from build123d import *

# Parameters (mm, degrees)
SKETCH1_R           = 2.5
BOSS_EXTRUDE1_DEPTH = 6


with BuildPart() as part:
    # Sketch1 → Boss-Extrude1 (new body)
    with BuildSketch(Plane(origin=(0, 0, 0), x_dir=(1, 0, 0), z_dir=(0, 1, 0))):
        with BuildLine():
            Line((29.312544284, -14.726094949), (29.830902437, -13.828272291))
            ThreePointArc((29.830902437, -13.828272291), (29.893839703, -13.350216293), (29.600306432, -12.967676287))
            Line((29.600306432, -12.967676287), (7.429695757, -0.167468245))
            ThreePointArc((7.429695757, -0.167468245), (7.128219563, -0.042592717), (6.804695757, 0))
            Line((6.804695757, 0), (-20.369097563, 0))
            ThreePointArc((-20.369097563, 0), (-21.25298104, -0.366116524), (-21.619097563, -1.25))
            Line((-21.619097563, -1.25), (-21.619097563, -23.75))
            ThreePointArc((-21.619097563, -23.75), (-21.25298104, -24.633883476), (-20.369097563, -25))
            Line((-20.369097563, -25), (-4.014034054, -25))
            ThreePointArc((-4.014034054, -25), (-3.690510247, -25.042592717), (-3.389034054, -25.167468245))
            Line((-3.389034054, -25.167468245), (16.070306432, -36.402323713))
            ThreePointArc((16.070306432, -36.402323713), (16.548362431, -36.465260979), (16.930902437, -36.171727709))
            Line((16.930902437, -36.171727709), (17.44926059, -35.273905051))
            ThreePointArc((17.44926059, -35.273905051), (17.815716934, -34.984910861), (18.280480237, -35.027372208))
            ThreePointArc((18.280480237, -35.027372208), (33.123688229, -30.625), (29.514650402, -15.569218702))
            ThreePointArc((29.514650402, -15.569218702), (29.245496145, -15.187952547), (29.312544284, -14.726094949))
        make_face()
        with Locations(Location((-14.119097563, -18.75, 0), (0, 0, 270))):
            Circle(SKETCH1_R, mode=Mode.SUBTRACT)
        with Locations(Location((-14.119097563, -6.25, 0), (0, 0, 90))):
            Circle(SKETCH1_R, mode=Mode.SUBTRACT)
        with BuildLine():
            Line((25.255902437, -21.752404736), (12.26552138, -14.252404736))
            ThreePointArc((12.26552138, -14.252404736), (7.142926116, -15.625), (8.51552138, -20.747595264))
            Line((8.51552138, -20.747595264), (21.505902437, -28.247595264))
            ThreePointArc((21.505902437, -28.247595264), (26.628497701, -26.875), (25.255902437, -21.752404736))
        make_face(mode=Mode.SUBTRACT)
    extrude(amount=BOSS_EXTRUDE1_DEPTH)


solid = part.part
Work out the finished part from the listing and answer in its coordinate system (mm). A direction names the side the tool comes from. Give positions to 0.01 mm unless a question says otherwise; leave off trailing zeros. Write each loop counter-clockwise with the first axis right and the second up, starting at its lowest first coordinate (ties: lowest second). Pieces come first, ordered by that corner, then holes. Notation, with made-up numbers: M 6,-24 L 30,-24 A17 ccw 30,-6 Z; hole C -18.75,76.5 d10. An arc over 180 degrees is marked long. Answer as CSV lines item,"result".
Q1. A cutting plane is placed at A-A on z = 26. Write down the section's boundary in (x, y).
A:
outline,"M -1.95,0 L 17.61,0 L 17.61,6 L -1.95,6 Z; M 27,0 L 34.59,0 L 34.59,6 L 27,6 Z"
Q2. Given P1, Ø4, axis at x = 26.5, z = 24, coming from the -Y side; P2, Ø3, axis at x = -12, y = 3.5, coming from the +Z side; P3, Ø3, axis at x = -14.12, z = 6.25, coming from the +Y side; P4, Ø1, axis at x = 24, y = 2.5, coming from the -Z side, each flat-ended and moving along its own axis, determine where each tip first touches the part or whether it passes through.
A:
P1,"stops at y = 0"
P2,"stops at z = 25"
P3,"passes through"
P4,"stops at z = 9.45"
Q3. A cutting plane is placed at D-D on z = 17.5. Write down the section's boundary in (x, y), plus the area to 3 significant figures.
A:
outline,"M -21.62,0 L -16.28,0 L -16.28,6 L -21.62,6 Z; M -11.95,0 L 6.64,0 L 6.64,6 L -11.95,6 Z; M 17.89,0 L 31.77,0 L 31.77,6 L 17.89,6 Z"
area,"227 mm²"
Q4. A cutting plane is placed at C-C on y = 2.15. Write down the section's boundary in (x, z), plus the area to 3 significant figures.
A:
outline,"M -21.62,1.25 A1.25 ccw -20.37,0 L 6.8,0 A1.25 ccw 7.43,0.17 L 29.6,12.97 A0.63 ccw 29.83,13.83 L 29.31,14.73 A0.63 cw 29.51,15.57 A11.25 ccw 18.28,35.03 A0.63 cw 17.45,35.27 L 16.93,36.17 A0.63 ccw 16.07,36.4 L -3.39,25.17 A1.25 cw -4.01,25 L -20.37,25 A1.25 ccw -21.62,23.75 Z; hole C -14.12,6.25 d5; hole C -14.12,18.75 d5; hole M 8.52,20.75 A3.75 ccw 12.27,14.25 L 25.26,21.75 A3.75 ccw 21.51,28.25 Z"
area,"1,260 mm²"
Q5. A cutting plane is placed at B-B on x = 22.5. Write down the section's boundary in (y, z).
A:
outline,"M 0,8.87 L 6,8.87 L 6,20.16 L 0,20.16 Z; M 0,28.65 L 6,28.65 L 6,36.22 L 0,36.22 Z"
Q6. The mould has two halves that part along Z. Classify faces 1 (the cylindrical face through (26.586, 2.958, 26.946)), 2 (the cylindrical face through (-21.263, 2.958, 24.624)), 3 (the flat face through (6, 0, 18)): +Z half, -Z half, draft (parallel to the pull), parting line (faces both ways), or undercut.
A:
face 1,"undercut"
face 2,"+Z half"
face 3,"draft"
Q7. A tool of negligible diameter and unlimited length cuts with its end or side. For faces 4 (the flat face through (-12, 3, 25)), 5 (the cylindrical face through (-21.243, 2.958, 0.356)), 6 (the flat face through (14.92, 2.958, 24.445)), from which of +Z, -Z, +X, -X, +Y, -Y can it reach the whole face along a straight path? Write none if from no direction.
A:
face 4,"+Z, -X, +Y, -Y"
face 5,"-Z, -X, +Y, -Y"
face 6,"+Y, -Y"
Q8. Find the intervals of material crossed by probe 1 along Z at (x, y) = (-14, 4.9); probe 2 along X at (y, z) = (2.2, 18); probe 3 along X at (y, z) = (4.1, 18.75), in increasing order. Write a range as [from, to].
A:
probe 1,"z = [0, 3.75], [8.75, 16.25], [21.25, 25]"
probe 2,"x = [-21.62, -16.5], [-11.73, 6.67], [18.76, 32.19]"
probe 3,"x = [-21.62, -16.62], [-11.62, 6.85], [20.06, 32.74]"
